```python
from build123d import *

# Parameters (mm, degrees)
F0_W           = 36
F0_H           = 3
F1_DEPTH       = 30
F0_H_2         = 27
F2_DEPTH       = 3
F4_D           = 3.4
F4_CSINK_D     = 6.72
F4_CSINK_ANGLE = 90
F5_D           = 3.3


with BuildPart() as f1:
    # F0 (on Front) → F1 (new body)
    with BuildSketch(Plane.XZ):
        with Locations((-9.6957933456, 0.646031009)):
            Rectangle(F0_W, F0_H)
    extrude(amount=F1_DEPTH)

    # F0 (on Front) → F2 (join)
    with BuildSketch(Plane.XZ):
        with Locations((-9.6957933456, 15.646031009)):
            Rectangle(F0_W, F0_H_2)
        with Locations((-9.6957933456, 0.646031009)):
            Rectangle(F0_W, F0_H)
    extrude(amount=F2_DEPTH)

    # F4 (through all)
    with Locations(Plane.XY.offset(2.146031009)):
        with Locations((-19.6957933456, -16.5), (0.3042066544, -16.5)):
            CounterSinkHole(F4_D / 2, F4_CSINK_D / 2, counter_sink_angle=F4_CSINK_ANGLE)

    # F5 (through all)
    with Locations(Plane(origin=(0, 0, 0), x_dir=(1, 0, 0), z_dir=(0, 1, 0))):
        with Locations((-9.6957933456, -15.146031009)):
            Hole(F5_D / 2)


solid = f1.part
```
Could you check a few things on this model? Use its own coordinates, in mm. Coordinates: 2 decimals unless noted, no trailing zeros. Order: outer loops, then holes, each group sorted by start corner. A loop starts at its lowest first (then second) coordinate and runs counter-clockwise, first axis right, second up. Notation, with made-up numbers: M -12,70.5 L 3,70.5 A33 cw 3,101.5 Z; hole C -15,-15 d3. An arc over 180 degrees is marked long. Use a Markdown table: item, result. Add a question column.
Q1. I want a section at B-B on z = 1.5. List the corners of the cut face in (x, y) for me, then the cut area to 3 significant figures.
Q2. I want a section at A-A on y = -16.5. List the corners of the cut face in (x, z) for me.
Q3. We'd pull the mould along Y, two halves only. Please class faces 1 (the flat face through (-10, -16, 2.146)), 2 (the cylindrical face through (-18.347, -17.534, -0.193)), 3 (the flat face through (-10, -3, 13)): pulls with the +Y half, pulls with the -Y half, needs draft (parallel to the pull), parting line crosses it, or undercut.
Q4. I want a section at C-C on x = -25. List the corners of the cut face in (y, z) for me.
Q5. I'm going to push flat-ended pins straight in: pin 1 (1 mm diameter, centred on x = -23, y = -15.5, fed in from +Z); pin 2 (10 mm diameter, centred on y = -6.5, z = 8.5, fed in from -X); pin 3 (3 mm diameter, centred on x = -19.7, y = -16.5, fed in from +Z); pin 4 (8 mm diameter, centred on x = -17.5, z = 15, fed in from -Y). Where does each tip first touch, or does it pass through?
Q6. I want a section at D-D on y = -21.5. List the corners of the cut face in (x, z) for me, then the cut area to 3 significant figures.
Q7. If I drill on L1, parallel to X at y = -16.5, z = -0.2; L2, parallel to Z at x = 5.5, y = -23.5; L3, parallel to Y at x = -26, z = 3.75, over which ranges is the centre line in solid material (lowest first)?
Checked values:
| question | item | result |
|---|---|---|
| 1 | outline | M -27.7,-30 L 8.3,-30 L 8.3,0 L -27.7,0 Z; hole C -19.7,-16.5 d5.43; hole C 0.3,-16.5 d5.43 |
| 1 | area | 1,030 mm² |
| 2 | outline | M -27.7,-0.85 L -21.4,-0.85 L -21.4,0.49 L -23.06,2.15 L -27.7,2.15 Z; M -18,-0.85 L -1.4,-0.85 L -1.4,0.49 L -3.06,2.15 L -16.34,2.15 L -18,0.49 Z; M 2,-0.85 L 8.3,-0.85 L 8.3,2.15 L 3.66,2.15 L 2,0.49 Z |
| 3 | face 1 | needs draft |
| 3 | face 2 | undercut |
| 3 | face 3 | pulls with the -Y half |
| 4 | outline | M -30,-0.85 L 0,-0.85 L 0,29.15 L -3,29.15 L -3,2.15 L -30,2.15 Z |
| 5 | pin 1 | z = 2.15 |
| 5 | pin 2 | x = -27.7 |
| 5 | pin 3 | through |
| 5 | pin 4 | y = -3 |
| 6 | outline | M -27.7,-0.85 L 8.3,-0.85 L 8.3,2.15 L -27.7,2.15 Z |
| 6 | area | 108 mm² |
| 7 | L1 | -27.7 to -21.4, -18 to -1.4, 2 to 8.3 |
| 7 | L2 | -0.85 to 2.15 |
| 7 | L3 | -3 to 0 |
